from build123d import *

# Parameters (mm, degrees)
BOSS_EXTRUDE1_DEPTH      = 4.5
BOSS_EXTRUDE1_DEPTH_BACK = 4.5
SKETCH1_R                = 33.725
CAVITY1_START            = 20.155580463
CAVITY1_OUTLINE_R        = 8.225
CAVITY1_DEPTH            = 4.5
CAVITY1_2_OUTLINE_R      = 9.725
CAVITY1_2_OUTLINE_R_2    = 8.225
CAVITY1_2_DEPTH          = 1.5
CAVITY1_START_2          = 23.155580463
CAVITY1_3_OUTLINE_R      = 9.725
CAVITY1_3_OUTLINE_R_2    = 8.225
CAVITY1_3_DEPTH          = 1.5
CAVITY1_START_3          = 17.905580463
CAVITY1_4_OUTLINE_R      = 3.725
CAVITY1_4_DEPTH          = 2.25
CAVITY1_5_DEPTH          = 2.25
CUT_EXTRUDE1_START       = 2.25
SKETCH1_3_R              = 9.725
CUT_EXTRUDE1_DEPTH       = 2.25
CUT_EXTRUDE2_DEPTH       = 2.25


with BuildPart() as part:
    # Sketch1 → Boss-Extrude1 (new, two sides: drawn at the far end of the back side and taken through both)
    with BuildSketch(Plane.XY.offset(22.405580463).offset(-BOSS_EXTRUDE1_DEPTH_BACK)):
        with Locations((-2.139643456, 12.812935379)):
            Circle(SKETCH1_R)
    extrude(amount=BOSS_EXTRUDE1_DEPTH + BOSS_EXTRUDE1_DEPTH_BACK)

    # Cavity1: read off the stored shape, not the designer's step
    # Cavity1 outline → Cavity1 (cut)
    with BuildSketch(Plane.XY.offset(CAVITY1_START)):
        with Locations((-2.139643456, 12.812935379)):
            Circle(CAVITY1_OUTLINE_R)
    extrude(amount=CAVITY1_DEPTH, mode=Mode.SUBTRACT)

    # Cavity1 2 outline → Cavity1 2 (cut)
    with BuildSketch(Plane.XY.offset(CAVITY1_START)):
        with Locations((-2.139643456, 12.812935379)):
            Circle(CAVITY1_2_OUTLINE_R)
        with Locations((-2.139643456, 12.812935379)):
            Circle(CAVITY1_2_OUTLINE_R_2, mode=Mode.SUBTRACT)
    extrude(amount=CAVITY1_2_DEPTH, mode=Mode.SUBTRACT)

    # Cavity1 3 outline → Cavity1 3 (cut)
    with BuildSketch(Plane.XY.offset(CAVITY1_START_2)):
        with Locations((-2.139643456, 12.812935379)):
            Circle(CAVITY1_3_OUTLINE_R)
        with Locations((-2.139643456, 12.812935379)):
            Circle(CAVITY1_3_OUTLINE_R_2, mode=Mode.SUBTRACT)
    extrude(amount=CAVITY1_3_DEPTH, mode=Mode.SUBTRACT)

    # Cavity1 4 outline → Cavity1 4 (cut)
    with BuildSketch(Plane.XY.offset(CAVITY1_START_3)):
        with Locations((-2.139643456, 12.812935379)):
            Circle(CAVITY1_4_OUTLINE_R)
    extrude(amount=CAVITY1_4_DEPTH, mode=Mode.SUBTRACT)

    # Sketch1<3> → Cut-Extrude1 (cut)
    with BuildSketch(Plane.XY.offset(22.405580463).offset(CUT_EXTRUDE1_START)):
        with Locations((-2.139643456, 12.812935379)):
            Circle(SKETCH1_3_R)
    cut_extrude1 = extrude(amount=CUT_EXTRUDE1_DEPTH, mode=Mode.SUBTRACT)

    # Mirror1: Cut-Extrude1 across plane
    add(cut_extrude1.mirror(Plane.XY.offset(22.405580463)), mode=Mode.SUBTRACT)


with BuildPart() as body_2:
    # Cavity1 5 outline → Cavity1 5 (new body)
    with BuildSketch(Plane.XY.offset(CAVITY1_START_3)):
        with BuildLine():
            ThreePointArc((-4.026439682, 14.637935379), (-4.764643456, 12.812935379), (-4.026439682, 10.987935379))
            Line((-4.026439682, 10.987935379), (-0.252847229, 10.987935379))
            ThreePointArc((-0.252847229, 10.987935379), (0.485356544, 12.812935379), (-0.252847229, 14.637935379))
            Line((-0.252847229, 14.637935379), (-4.026439682, 14.637935379))
        make_face()
    extrude(amount=CAVITY1_5_DEPTH)

    # Sketch2 → Cut-Extrude2 (cut)
    with BuildSketch(Plane.XY.offset(20.155580463)):
        with BuildLine():
            Line((-0.252847229, 14.637935379), (-4.026439682, 14.637935379))
            ThreePointArc((-4.026439682, 14.637935379), (-4.764643456, 12.812935379), (-4.026439682, 10.987935379))
            Line((-4.026439682, 10.987935379), (-0.252847229, 10.987935379))
            ThreePointArc((-0.252847229, 10.987935379), (0.485356544, 12.812935379), (-0.252847229, 14.637935379))
        make_face()
    extrude(amount=-CUT_EXTRUDE2_DEPTH, mode=Mode.SUBTRACT)


solid = part.part
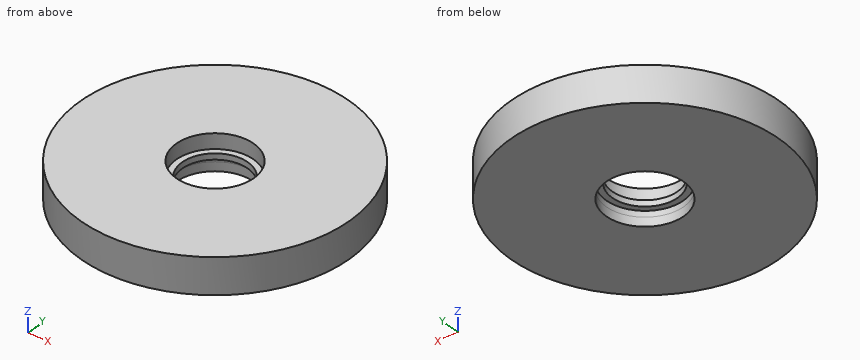
For this review, take the finished solid that the model builds, in its own axes (mm). Give positions to 0.01 mm unless a question says otherwise; leave off trailing zeros. Loops run counter-clockwise (first coordinate to the right, second up) from the corner with the lowest first, then second, coordinate; pieces in that order, holes last. Notation, with made-up numbers: M 25,-19 L 77,-19 A25 ccw 77,9 Z; hole C 62.25,29.5 d9. An arc over 180 degrees is marked long. Put each result on its own line as item: value. Start each with the question number.
(1) Wall thickness on L1, parallel to Y at x = -2.5, z = 20.25; L2, parallel to X at y = 8.5, z = 26; L3, parallel to Y at x = 0, z = 19.5: over which ranges is each line inside the solid? List them lowest first.
(2) Add section C-C, the plane z = 24.75. Write out the cut boundary in (x, y) (3 decimals).
(3) Add section B-B, the plane y = 12. Write out the cut boundary in (x, z).
(4) Add section A-A, the plane x = -8. Write out the cut boundary in (y, z).
(5) Add section D-D, the plane y = 1.5. Write out the cut boundary in (x, z).
(6) For pin 1 (1.5 mm diameter, centred on y = 23.5, z = 19, fed in from +X); pin 2 (2 mm diameter, centred on y = 39.5, z = 26, fed in from -X); pin 3 (11.5 mm diameter, centred on x = -2.14, y = 12.81, fed in from -Z); pin 4 (5 mm diameter, centred on x = -3.5, z = 19.5, fed in from +Y), all flat-tipped, find the tip position at first contact; note any pin that passes through.
Result:
1. L1: y = -20.91 to 3.09, 22.53 to 46.54
1. L2: x = -35.59 to -10.86, 6.58 to 31.31
1. L3: y = -20.84 to 3.33, 22.3 to 46.47
2. outline: C -2.14,12.813 d67.45; hole C -2.14,12.813 d19.45
3. outline: M -35.85,17.91 L -11.83,17.91 L -11.83,21.66 L -10.32,21.66 L -10.32,23.16 L -11.83,23.16 L -11.83,26.91 L -35.85,26.91 Z; M 6.05,21.66 L 7.55,21.66 L 7.55,17.91 L 31.58,17.91 L 31.58,26.91 L 7.55,26.91 L 7.55,23.16 L 6.05,23.16 Z
4. outline: M -20.4,17.91 L 5.05,17.91 L 5.05,21.66 L 7.04,21.66 L 7.04,23.16 L 5.05,23.16 L 5.05,26.91 L -20.4,26.91 Z; M 18.58,21.66 L 20.57,21.66 L 20.57,17.91 L 46.02,17.91 L 46.02,26.91 L 20.57,26.91 L 20.57,23.16 L 18.58,23.16 Z
5. outline: M -33.91,17.91 L 29.63,17.91 L 29.63,26.91 L -33.91,26.91 Z
6. pin 1: stops at x = 30.09
6. pin 2: stops at x = -23.99
6. pin 3: passes through
6. pin 4: stops at y = 46.54
